Part model, mm, in its own coordinate system. A direction names the side the tool comes from. Coordinates: 2 decimals unless noted, no trailing zeros. Loops run counter-clockwise (first coordinate to the right, second up) from the corner with the lowest first, then second, coordinate; pieces in that order, holes last. Notation, with made-up numbers: M 13.5,79.5 L 32.5,79.5 A17 cw 32.5,100.5 Z; hole C 74.5,-33.5 d2. An arc over 180 degrees is marked long. Use CSV: the item, a comma, the result in double quotes. Start each with the question number.
from build123d import *

# Parameters (mm, degrees)
ESQUISSE1_R                  = 5.75
ESQUISSE1_R_2                = 1.6
BOSS_EXTRU_1_DEPTH           = 5
ESQUISSE2_R                  = 3
ENL_V_MAT_EXTRU_1_DEPTH      = 3
ENL_V_START                  = -3
ESQUISSE3_R                  = 5.75
ESQUISSE3_R_2                = 4.5
ENL_V_MAT_EXTRU_2_DEPTH      = 3
BOSS_EXTRU_2_DEPTH           = 2
R_P_TITION_CIRCULAIRE1_COUNT = 2
ESQUISSE5_R                  = 0.75
ENL_V_MAT_EXTRU_3_DEPTH      = 3
R_P_TITION_CIRCULAIRE2_COUNT = 2
BOSS_EXTRU_3_DEPTH           = 3
R_P_TITION_CIRCULAIRE3_COUNT = 28
ENL_V_START_2                = -1
ESQUISSE7_R                  = 3
ESQUISSE7_R_2                = 1.6
ENL_V_MAT_EXTRU_4_DEPTH      = 1
ESQUISSE8_R                  = 4.7
ESQUISSE8_R_2                = 3.4
ENL_V_MAT_EXTRU_5_DEPTH      = 1
SKETCH1_R                    = 0.75
CUT_EXTRUDE1_DEPTH           = 10


with BuildPart() as part:
    # Esquisse1 → Boss.-Extru.1 (new body)
    with BuildSketch(Plane.XY):
        Circle(ESQUISSE1_R)
        Circle(ESQUISSE1_R_2, mode=Mode.SUBTRACT)
    extrude(amount=BOSS_EXTRU_1_DEPTH)

    # Esquisse2 → Enlèv. mat.-Extru.1 (cut)
    with BuildSketch(Plane.XY.offset(5)):
        Circle(ESQUISSE2_R)
    extrude(amount=-ENL_V_MAT_EXTRU_1_DEPTH, mode=Mode.SUBTRACT)

    # Esquisse3 → Enlèv. mat.-Extru.2 (cut)
    with BuildSketch(Plane.XY.offset(5).offset(ENL_V_START)):
        Circle(ESQUISSE3_R)
        Circle(ESQUISSE3_R_2, mode=Mode.SUBTRACT)
    extrude(amount=ENL_V_MAT_EXTRU_2_DEPTH, mode=Mode.SUBTRACT)

    # Esquisse4 → Boss.-Extru.2 (add)
    with BuildSketch(Plane(origin=(0, 0, 0), x_dir=(-1, 0, 0), z_dir=(0, 0, -1))):
        with BuildLine():
            Line((-4.3, 3.817394399), (-2.475852955, 16.846629695))
            ThreePointArc((-2.475852955, 16.846629695), (0, 19), (2.475852955, 16.846629695))
            Line((2.475852955, 16.846629695), (4.3, 3.817394399))
            ThreePointArc((4.3, 3.817394399), (0, 5.75), (-4.3, 3.817394399))
        make_face()
    boss_extru_2 = extrude(amount=-BOSS_EXTRU_2_DEPTH)

    # Répétition circulaire1: Boss.-Extru.2 ×2 about axis
    r_p_tition_circulaire1_axis = Axis((0, 0, 0), (0, 0, 1))
    for i in range(1, R_P_TITION_CIRCULAIRE1_COUNT):
        add(boss_extru_2.rotate(r_p_tition_circulaire1_axis, i * 360 / R_P_TITION_CIRCULAIRE1_COUNT))

    # Esquisse5 → Enlèv. mat.-Extru.3 (cut)
    with BuildSketch(Plane(origin=(0, 0, 0), x_dir=(-1, 0, 0), z_dir=(0, 0, -1))):
        with Locations((0, 7)):
            Circle(ESQUISSE5_R)
        with Locations((0, 10)):
            Circle(ESQUISSE5_R)
        with Locations((0, 13)):
            Circle(ESQUISSE5_R)
        with Locations((0, 16)):
            Circle(ESQUISSE5_R)
    enl_v_mat_extru_3 = extrude(amount=-ENL_V_MAT_EXTRU_3_DEPTH, mode=Mode.SUBTRACT)

    # Répétition circulaire2: Enlèv. mat.-Extru.3 ×2 about axis
    r_p_tition_circulaire2_axis = Axis((0, 0, 0), (0, 0, 1))
    for i in range(1, R_P_TITION_CIRCULAIRE2_COUNT):
        add(enl_v_mat_extru_3.rotate(r_p_tition_circulaire2_axis, i * 360 / R_P_TITION_CIRCULAIRE2_COUNT), mode=Mode.SUBTRACT)

    # Esquisse6 → Boss.-Extru.3 (add)
    with BuildSketch(Plane.XY.offset(5)):
        Polygon((-0.3, 3), (0, 2.7), (0.3, 3), align=None)
    boss_extru_3 = extrude(amount=-BOSS_EXTRU_3_DEPTH)

    # Répétition circulaire3: Boss.-Extru.3 ×28 about axis
    r_p_tition_circulaire3_axis = Axis((0, 0, 0), (0, 0, 1))
    for i in range(1, R_P_TITION_CIRCULAIRE3_COUNT):
        add(boss_extru_3.rotate(r_p_tition_circulaire3_axis, i * 360 / R_P_TITION_CIRCULAIRE3_COUNT))

    # Esquisse7 → Enlèv. mat.-Extru.4 (cut)
    with BuildSketch(Plane(origin=(0, 0, 0), x_dir=(-1, 0, 0), z_dir=(0, 0, -1)).offset(ENL_V_START_2)):
        Circle(ESQUISSE7_R)
        Circle(ESQUISSE7_R_2, mode=Mode.SUBTRACT)
    extrude(amount=ENL_V_MAT_EXTRU_4_DEPTH, mode=Mode.SUBTRACT)

    # Esquisse8 → Enlèv. mat.-Extru.5 (cut)
    with BuildSketch(Plane(origin=(0, 0, 0), x_dir=(-1, 0, 0), z_dir=(0, 0, -1))):
        Circle(ESQUISSE8_R)
        Circle(ESQUISSE8_R_2, mode=Mode.SUBTRACT)
    extrude(amount=-ENL_V_MAT_EXTRU_5_DEPTH, mode=Mode.SUBTRACT)

    # Sketch1 → Cut-Extrude1 (cut)
    with BuildSketch(Plane(origin=(0, 0, 0), x_dir=(-1, 0, 0), z_dir=(0, 0, -1))):
        with BuildLine():
            Line((-2.475852955, 16.846629695), (-4.3, 3.817394399))
            ThreePointArc((-4.3, 3.817394399), (0, 5.75), (4.3, 3.817394399))
            Line((4.3, 3.817394399), (2.475852955, 16.846629695))
            ThreePointArc((2.475852955, 16.846629695), (0, 19), (-2.475852955, 16.846629695))
        make_face()
        with Locations((0, 7)):
            Circle(SKETCH1_R, mode=Mode.SUBTRACT)
        with Locations((0, 10)):
            Circle(SKETCH1_R, mode=Mode.SUBTRACT)
        with Locations((0, 13)):
            Circle(SKETCH1_R, mode=Mode.SUBTRACT)
        with Locations((0, 16)):
            Circle(SKETCH1_R, mode=Mode.SUBTRACT)
    extrude(amount=-CUT_EXTRUDE1_DEPTH, mode=Mode.SUBTRACT)


solid = part.part
1. Wall check: probe 1 along X at (y, z) = (0, 1.4); probe 2 along X at (y, z) = (1, 0.9); probe 3 along X at (y, z) = (2, 0.75). Give the ranges that are in metal, low to high.
2. Slice it at D-D, the plane x = -5. List the corners of the cut face in (y, z).
3. Two-plate mould, pull along X, no slides. Class faces 4 (the face through (0, -19, 1)), 5 (the face through (-0.163, -15.268, 0.986)), 6 (the face through (-3.4, -10.24, 0.99)), 7 (the face through (-1, -6, 2)): pulls with the +X half, pulls with the -X half, needs draft (parallel to the pull), parting line crosses it, or undercut.
4. Slice it at B-B, the plane y = -13. List the corners of the cut face in (x, z).
5. Tool access for faces 1 (the face through (-0.59, 4.46, 3.48)), 2 (the face through (-0.098, -13.744, 0.986)), 3 (the face through (0.74, -3.32, 0.49)): list every direction of +Z, -Z, +X, -X, +Y, -Y with a clear straight run to the whole face (end or side of a thin tool).
6. Pin check, flat tips, straight feed: pin 1 (2.5 mm diameter, centred on x = 0, y = -10, fed in from +Z); pin 2 (1.5 mm diameter, centred on x = 0, z = 4.5, fed in from -Y); pin 3 (2.5 mm diameter, centred on x = 0, y = 0, fed in from +Z); pin 4 (1.8 mm diameter, centred on x = -1, y = -1, fed in from -Z). Stop position of each tip, or through.
7. Slice it at A-A, the plane z = 1.6. List the corners of the cut face in (x, y), and give its area (3 significant figures).
8. Slice it at C-C, the plane y = -7. List the corners of the cut face in (x, z).
Found:
1,probe 1,"-5.75 to -1.6, 1.6 to 5.75"
1,probe 2,"-5.66 to -4.59, -3.25 to -2.83, 2.83 to 3.25, 4.59 to 5.66"
1,probe 3,"-5.39 to -4.25, -2.75 to -2.24, 2.24 to 2.75, 4.25 to 5.39"
2,outline,"M -2.84,0 L 2.84,0 L 2.84,2 L -2.84,2 Z"
3,face 4,"parting line crosses it"
3,face 5,"undercut"
3,face 6,"pulls with the -X half"
3,face 7,"needs draft"
4,outline,"M -3.01,0 L -0.75,0 L -0.75,2 L -3.01,2 Z; M 0.75,0 L 3.01,0 L 3.01,2 L 0.75,2 Z"
5,face 1,"+Z"
5,face 2,"+Z, -Z"
5,face 3,"-Z"
6,pin 1,"z = 2"
6,pin 2,"y = -4.5"
6,pin 3,"through"
6,pin 4,"z = 1"
7,outline,"M -4.3,-3.82 L -2.48,-16.85 A2.5 ccw 2.48,-16.85 L 4.3,-3.82 A5.75 ccw long Z; hole C 0,0 d3.2; hole C 0,-16 d1.5; hole C 0,-13 d1.5; hole C 0,-10 d1.5; hole C 0,-7 d1.5"
7,area,"174 mm^2"
8,outline,"M -3.85,0 L -0.75,0 L -0.75,2 L -3.85,2 Z; M 0.75,0 L 3.85,0 L 3.85,2 L 0.75,2 Z"
